Work out the finished part from the listing and answer in its coordinate system (mm). Face numbers are marked on the shaded views. A direction names the side the tool comes from. Coordinates: 2 decimals unless noted, no trailing zeros. Loops run counter-clockwise (first coordinate to the right, second up) from the corner with the lowest first, then second, coordinate; pieces in that order, holes last. Notation, with made-up numbers: (20, 36.25) - (79, 36.25) arc R18 ccw to (79, 47.25) - close; hole circle Ø3 at (21, 51.25). An arc over 180 degrees is marked (long way). Write each question's results on one line, items separated by ' | '. Start each with the question number.
Item 1: Each of these flat-tipped pins is pushed along its axis until it touches: pin 1 Ø5 at (x, z) = (5, 9) entering from +Y; pin 2 Ø7 at (x, y) = (-28, 1.5) entering from +Z; pin 3 Ø1.5 at (y, z) = (-18, 3) entering from -X; pin 4 Ø3 at (y, z) = (-16, 8.5) entering from +X. Where does it stop, or does it pass through?
Item 2: A tool of negligible diameter and unlimited length cuts with its end or side. For the marked faces 4, 5 and 6, from which of +Z, -Z, +X, -X, +Y, -Y can it reach the whole face along a straight path? Write none if from no direction.
Item 3: For a pull along X with two mould halves and no side action, classify the marked faces 1, 2 and 3 as +X half, -X half, draft (parallel to the pull), parting line (faces both ways), or undercut.
Item 4: Consider probe 1 along Y at (x, z) = (-28.5, 2); probe 2 along X at (y, z) = (-11.5, 7.5); probe 3 along Y at (x, z) = (26.5, 10.5). Determine where each line is inside the solid, lowest interval first. Write a range as [from, to].
Item 5: Section A-A, the plane y = -14.5 is taken. Write down the section's boundary in (x, z), plus the area to 3 significant figures.
Item 6: Section D-D, the plane x = -21 is taken. Write down the section's boundary in (y, z), plus the area to 3 significant figures.
Item 7: Section B-B, the plane z = 1 is taken. Write down the section's boundary in (x, y).
Item 8: Section C-C, the plane y = -6.5 is taken. Write down the section's boundary in (x, z), plus the area to 3 significant figures.
from build123d import *

# Parameters (mm, degrees)
BOSS_EXTRUDE8_DEPTH       = 12
SKETCH4_W                 = 8
SKETCH4_H                 = 4
BOSS_EXTRUDE10_DEPTH      = 12
SKETCH5_R                 = 1.5
CUT_EXTRUDE2_DEPTH        = 12
SKETCH6_W                 = 10
SKETCH6_H                 = 9
BOSS_EXTRUDE11_DEPTH      = 1
BOSS_EXTRUDE11_DEPTH_BACK = 5.8
SKETCH7_R                 = 1.5
CUT_EXTRUDE3_DEPTH        = 10
FILLET1_R                 = 3
FILLET3_R                 = 3
FILLET4_R                 = 3
FILLET5_R                 = 3
FILLET6_R                 = 3


with BuildPart() as part:
    # Sketch1 → Boss-Extrude8 (new body)
    with BuildSketch(Plane.XY):
        with BuildLine():
            Line((25, 0), (19.5, 0))
            ThreePointArc((19.5, 0), (0, -19.5), (-19.5, 0))
            Line((-19.5, 0), (-25, 0))
            ThreePointArc((-25, 0), (0, -25), (25, 0))
        make_face()
    extrude(amount=BOSS_EXTRUDE8_DEPTH)

    # Sketch4 → Boss-Extrude10 (add)
    with BuildSketch(Plane(origin=(0, 0, 0), x_dir=(-1, 0, 0), z_dir=(0, 0, -1))):
        with Locations((-27.5, -2)):
            Rectangle(SKETCH4_W, SKETCH4_H)
    extrude(amount=-BOSS_EXTRUDE10_DEPTH)

    # Sketch5 → Cut-Extrude2 (cut)
    with BuildSketch(Plane.XZ.offset(4)):
        with Locations((28.177925359, 6)):
            Circle(SKETCH5_R)
    extrude(amount=-CUT_EXTRUDE2_DEPTH, mode=Mode.SUBTRACT)

    # Sketch6 → Boss-Extrude11 (add, two sides)
    with BuildSketch(Plane(origin=(0, 0, 0), x_dir=(-1, 0, 0), z_dir=(0, 0, -1))) as boss_extrude11_sk:
        with Locations((27.5, 0)):
            Rectangle(SKETCH6_W, SKETCH6_H)
    extrude(amount=BOSS_EXTRUDE11_DEPTH)
    extrude(boss_extrude11_sk.sketch, amount=-BOSS_EXTRUDE11_DEPTH_BACK)

    # Sketch7 → Cut-Extrude3 (cut)
    with BuildSketch(Plane(origin=(0, 0, -1), x_dir=(-1, 0, 0), z_dir=(0, 0, -1))):
        with Locations((28.5, 0.5)):
            Circle(SKETCH7_R)
    extrude(amount=-CUT_EXTRUDE3_DEPTH, mode=Mode.SUBTRACT)

    # Fillet1
    fillet1_edges = [part.edges().sort_by_distance(p)[0] for p in [
        (-32.5, -4.5, 2.4),
    ]]
    fillet(fillet1_edges, radius=FILLET1_R)

    # Fillet3
    fillet3_edges = [part.edges().sort_by_distance(p)[0] for p in [
        (-32.5, 4.5, 2.4),
    ]]
    fillet(fillet3_edges, radius=FILLET3_R)

    # Fillet4
    fillet4_edges = [part.edges().sort_by_distance(p)[0] for p in [
        (-22.5, 4.5, 2.4),
    ]]
    fillet(fillet4_edges, radius=FILLET4_R)

    # Fillet5
    fillet5_edges = [part.edges().sort_by_distance(p)[0] for p in [
        (31.5, -2, 0),
    ]]
    fillet(fillet5_edges, radius=FILLET5_R)

    # Fillet6
    fillet6_edges = [part.edges().sort_by_distance(p)[0] for p in [
        (31.5, -2, 12),
    ]]
    fillet(fillet6_edges, radius=FILLET6_R)


solid = part.part
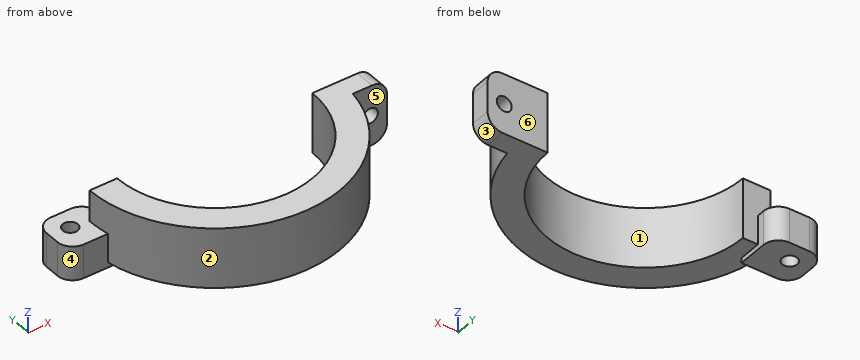
Answer key:
1) pin 1: stops at y = -18 | pin 2: stops at z = 12 | pin 3: stops at x = -18.1 | pin 4: stops at x = 20.37
2) face 4: +Z, -Z, -X, -Y | face 5: +Z, -Z, +X, -Y | face 6: +Z, -Z, +X, +Y
3) face 1: undercut | face 2: parting line | face 3: +X half
4) probe 1: y = [-4.5, -1], [2, 4.5] | probe 2: x = [-22.2, -15.75], [15.75, 22.2] | probe 3: y = [-4, 0]
5) outline: (-20.37, 0) - (-13.04, 0) - (-13.04, 12) - (-20.37, 12) - close; (13.04, 0) - (20.37, 0) - (20.37, 12) - (13.04, 12) - close | area: 176 mm^2
6) outline: (-13.56, 0) - (0, 0) - (0, 12) - (-13.56, 12) - close | area: 163 mm^2
7) outline: (-32.5, -1.5) arc R3 ccw to (-29.5, -4.5) - (-24.59, -4.5) arc R25 ccw to (24.68, -4) - (30.74, -4) - (30.74, 0) - (19.5, 0) arc R19.5 cw to (-19.5, 0) - (-22.5, 0) - (-22.5, 1.5) arc R3 ccw to (-25.5, 4.5) - (-29.5, 4.5) arc R3 ccw to (-32.5, 1.5) - close; hole circle Ø3 at (-28.5, 0.5)
8) outline: (-24.14, 0) - (-18.38, 0) - (-18.38, 12) - (-24.14, 12) - close; (18.38, 0) - (24.14, 0) - (24.14, 12) - (18.38, 12) - close | area: 138 mm^2
